from build123d import *

# Parameters (mm, degrees)
SCHIZZO1_R                   = 4
ESTRUSIONE_ESTRUSIONE1_DEPTH = 20
SMUSSO1_SIZE                 = 1
SCHIZZO6_R                   = 6.5
ESTRUSIONE_ESTRUSIONE3_DEPTH = 8
TAGLIO_ESTRUSIONE3_DEPTH     = 6
SCHIZZO8_R                   = 3.464101615
TAGLIO_ESTRUSIONE4_DEPTH     = 1
TAGLIO_ESTRUSIONE4_TAPER     = 45
RACCORDO1_R                  = 0.5
SCHIZZO9_R                   = 12
SCHIZZO9_R_2                 = 6.5
ESTRUSIONE_ESTRUSIONE4_DEPTH = 2
RACCORDO2_R                  = 0.1


with BuildPart() as part:
    # Schizzo1 → Estrusione-Estrusione1 (new body)
    with BuildSketch(Plane.XY):
        Circle(SCHIZZO1_R)
    extrude(amount=ESTRUSIONE_ESTRUSIONE1_DEPTH)

    # Smusso1
    smusso1_edges = [part.edges().sort_by_distance(p)[0] for p in [
        (-4, 0, 0),
    ]]
    chamfer(smusso1_edges, length=SMUSSO1_SIZE)

    # Schizzo6 → Estrusione-Estrusione3 (add)
    with BuildSketch(Plane.XY.offset(20)):
        Circle(SCHIZZO6_R)
    extrude(amount=ESTRUSIONE_ESTRUSIONE3_DEPTH)

    # Schizzo7 → Taglio-Estrusione3 (cut)
    with BuildSketch(Plane.XY.offset(28)):
        Polygon((1.732050808, 3), (-1.732050808, 3), (-3.464101615, 0), (-1.732050808, -3), (1.732050808, -3), (3.464101615, 0), align=None)
    extrude(amount=-TAGLIO_ESTRUSIONE3_DEPTH, mode=Mode.SUBTRACT)

    # Schizzo8 → Taglio-Estrusione4 (cut)
    with BuildSketch(Plane.XY.offset(28)):
        Circle(SCHIZZO8_R)
    extrude(amount=-TAGLIO_ESTRUSIONE4_DEPTH, taper=TAGLIO_ESTRUSIONE4_TAPER, mode=Mode.SUBTRACT)

    # Raccordo1
    raccordo1_edges = [part.edges().sort_by_distance(p)[0] for p in [
        (-6.5, 0, 28),
    ]]
    fillet(raccordo1_edges, radius=RACCORDO1_R)

    # Schizzo9 → Estrusione-Estrusione4 (add)
    with BuildSketch(Plane(origin=(0, 0, 20), x_dir=(-1, 0, 0), z_dir=(0, 0, -1))):
        Circle(SCHIZZO9_R)
        Circle(SCHIZZO9_R_2, mode=Mode.SUBTRACT)
    extrude(amount=-ESTRUSIONE_ESTRUSIONE4_DEPTH)

    # Raccordo2
    raccordo2_edges = [part.edges().sort_by_distance(p)[0] for p in [
        (-6.5, 0, 22),
        (12, 0, 22),
        (12, 0, 20),
    ]]
    fillet(raccordo2_edges, radius=RACCORDO2_R)


solid = part.part
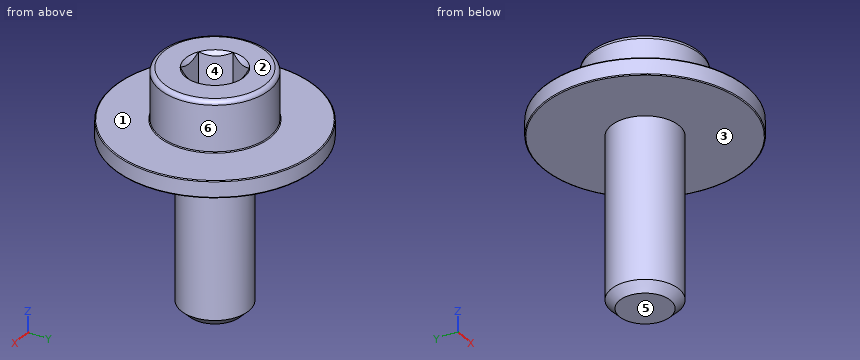
Geometry: final body of the model. Coordinates: model frame, mm. Face numbers are marked on the shaded views. A direction names the side the tool comes from. Coordinates: 2 decimals unless noted, no trailing zeros. Loops run counter-clockwise (first coordinate to the right, second up) from the corner with the lowest first, then second, coordinate; pieces in that order, holes last. Notation, with made-up numbers: M 22.25,-25.5 L 74.25,-25.5 A20 ccw 74.25,0.5 Z; hole C -13.75,18.25 d3. An arc over 180 degrees is marked long. One line per item, written item: value. Start each with the question number.
1) Pin query (flat end, axial travel): P1, Ø4, axis at x = 0, z = 25.5, coming from the -Y side; P2, Ø10, axis at x = -4, z = 3, coming from the +Y side; P3, Ø5, axis at y = -3.5, z = 11, coming from the -X side; P4, Ø3, axis at y = -6, z = 9, coming from the -X side. Return the tip coordinate at first contact, or that it passes through.
2) Draft query along Y for the marked faces 4, 5 and 6. Return one class per face: released by +Y, released by -Y, zero draft, split by the parting line, or undercut.
3) Reachability of the marked faces 1, 2 and 3 from +Z, -Z, +X, -X, +Y, -Y: full face, straight path, thin tool, end or side. Return the list, or none.
4) Cut plane A-A (z = 25.5). Return loops of the section in (x, y), then the cut area to 3 significant figures.
5) Cut plane C-C (z = 13.75). Return loops of the section in (x, y).
6) Material intervals for L1, parallel to Z at x = 1.75, y = -10; L2, parallel to X at y = -0.25, z = 22.25; L3, parallel to X at y = 1, z = 23.25, sorted ascending. Write a range as from..to.
7) Cut plane B-B (x = 0). Return loops of the section in (y, z), then the cut area to 3 significant figures.
Evaluation:
1. P1: y = -6.5
1. P2: y = 4
1. P3: x = -3.87
1. P4: through
2. face 4: undercut
2. face 5: zero draft
2. face 6: split by the parting line
3. face 1: +Z
3. face 2: +Z, +X, -X, +Y, -Y
3. face 3: -Z
4. outline: C 0,0 d13; hole M -3.46,0 L -1.73,-3 L 1.73,-3 L 3.46,0 L 1.73,3 L -1.73,3 Z
4. area: 102 mm^2
5. outline: C 0,0 d8
6. L1: 20..22
6. L2: -6.5..-3.32, 3.32..6.5
6. L3: -6.42..-2.89, 2.89..6.42
7. outline: M -12,20.1 A0.1 ccw -11.9,20 L -4,20 L -4,1 L -3,0 L 3,0 L 4,1 L 4,20 L 11.9,20 A0.1 ccw 12,20.1 L 12,21.9 A0.1 ccw 11.9,22 L 6.6,22 A0.1 cw 6.5,22.1 L 6.5,27.5 A0.5 ccw 6,28 L 3.46,28 L 3,27.54 L 3,22 L -3,22 L -3,27.54 L -3.46,28 L -6,28 A0.5 ccw -6.5,27.5 L -6.5,22.1 A0.1 cw -6.6,22 L -11.9,22 A0.1 ccw -12,21.9 Z
7. area: 249 mm^2
